from build123d import *

# Parameters (mm, degrees)
SKETCH_1_W      = 6
SKETCH_1_H      = 6
EXTRUDE_1_DEPTH = 2
SKETCH_3_W      = 8
SKETCH_3_H      = 8
EXTRUDE_2_DEPTH = 1
CHAMFER_1_SIZE  = 1


with BuildPart() as part:
    # 草图1 → 凸台-拉伸1 (new body)
    with BuildSketch(Plane(origin=(0, 0, 0), x_dir=(1, 0, 0), z_dir=(0, 1, 0))):
        Rectangle(SKETCH_1_W, SKETCH_1_H)
    extrude(amount=EXTRUDE_1_DEPTH)

    # 草图3 → 凸台-拉伸2 (add)
    with BuildSketch(Plane(origin=(0, 0, 0), x_dir=(1, 0, 0), z_dir=(0, 1, 0))):
        Rectangle(SKETCH_3_W, SKETCH_3_H)
    extrude(amount=EXTRUDE_2_DEPTH)

    # 倒角1
    chamfer_1_edges = [part.edges().sort_by_distance(p)[0] for p in [
        (0, 1, -4),
        (4, 1, 0),
        (0, 1, 4),
        (-4, 1, 0),
    ]]
    chamfer(chamfer_1_edges, length=CHAMFER_1_SIZE - 0.0001)  # a hair under: the kernel refuses the full size


solid = part.part
Here's how the part is built. I have some questions about the finished solid (model axes, mm). A direction names the side the tool comes from. Round coordinates to 2 decimals unless told otherwise and drop trailing zeros. Order: outer loops, then holes, each group sorted by start corner. A loop starts at its lowest first (then second) coordinate and runs counter-clockwise, first axis right, second up. Notation, with made-up numbers: M -17,-40 L 24,-40 A23 cw 24,-16 Z; hole C -11,30.25 d8. An arc over 180 degrees is marked long. Return JSON: item names as keys, results as strings. Group by question number.
1. On a 3-axis mill with a long thin cutter (end or side, diameter ignored), from which of +Z, -Z, +X, -X, +Y, -Y can I reach the whole of each face in a straight line? I mean faces 1 (the face through (3, 1.5, 0)), 2 (the face through (-3, 1.5, 0)), 3 (the face through (0, 1.5, -3)), 4 (the face through (0, 1.5, 3)). Say none if no direction works.
2. If we section it at C-C on y = 1.85: List the corners of the cut face in (x, z) for me.
3. Please list where these lines run through material, in increasing order: probe 1 along Z at (x, y) = (-2, 1.6); probe 2 along Z at (x, y) = (-0.75, 0.65).
4. I'm going to push flat-ended pins straight in: pin 1 Ø1.1 at (x, y) = (1, 1.5) entering from +Z; pin 2 Ø0.5 at (y, z) = (1.5, -0.5) entering from -X; pin 3 Ø4 at (x, z) = (-2, -2) entering from -Y; pin 4 Ø0.5 at (x, y) = (0, 1.5) entering from -Z. Where does each tip first touch, or does it pass through?
Reply:
{
 "1": {"face 1": "+Z, -Z, +X, +Y", "face 2": "+Z, -Z, -X, +Y", "face 3": "-Z, +X, -X, +Y", "face 4": "+Z, +X, -X, +Y"},
 "2": {"outline": "M -3,-3 L 3,-3 L 3,3 L -3,3 Z"},
 "3": {"probe 1": "-3 to 3", "probe 2": "-3.35 to 3.35"},
 "4": {"pin 1": "z = 3.05", "pin 2": "x = -3", "pin 3": "y = 0", "pin 4": "z = -3"}
}
